Geometry: final body of the model. Coordinates: model frame, mm. Give positions to 0.01 mm unless a question says otherwise; leave off trailing zeros. Write each loop counter-clockwise with the first axis right and the second up, starting at its lowest first coordinate (ties: lowest second). Pieces come first, ordered by that corner, then holes.
```python
from build123d import *

# Parameters (mm, degrees)
BOSS_EXTRUDE1_DEPTH = 5
SKETCH2_W           = 10
SKETCH2_H           = 4
BOSS_EXTRUDE2_DEPTH = 80
FILLET1_R           = 10


with BuildPart() as part:
    # Sketch1 → Boss-Extrude1 (new, symmetric)
    with BuildSketch(Plane(origin=(0, 0, 0), x_dir=(0, 0, -1), z_dir=(1, 0, 0))):
        with BuildLine():
            Line((-75.25, 40), (160.25, 40))
            ThreePointArc((160.25, 40), (166.57455532, 38.973665961), (172.25, 36))
            Line((172.25, 36), (-87.25, 36))
            ThreePointArc((-87.25, 36), (-81.57455532, 38.973665961), (-75.25, 40))
        make_face()
    extrude(amount=BOSS_EXTRUDE1_DEPTH, both=True)

    # Sketch2 → Boss-Extrude2 (add, symmetric)
    with BuildSketch(Plane(origin=(0, 0, 0), x_dir=(0, 0, -1), z_dir=(1, 0, 0))):
        with Locations((42.5, 38)):
            Rectangle(SKETCH2_W, SKETCH2_H)
    extrude(amount=BOSS_EXTRUDE2_DEPTH, both=True)

    # Fillet1
    fillet1_edges = [part.edges().sort_by_distance(p)[0] for p in [
        (-5, 38, -47.5),
        (-5, 38, -37.5),
        (5, 38, -37.5),
        (5, 38, -47.5),
    ]]
    fillet(fillet1_edges, radius=FILLET1_R)


solid = part.part
```
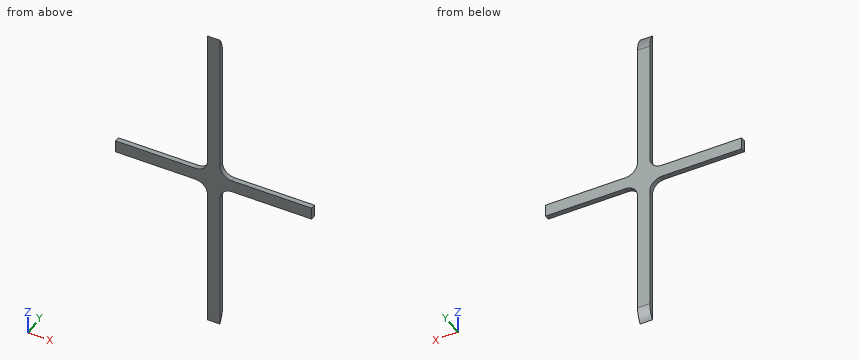
Item 1: Section A-A, the plane y = 36.9. Return the cut outline in (x, z).
Found:
outline: (-80, -47.5) - (-15, -47.5) arc R10 cw to (-5, -57.5) - (-5, -170.95) - (5, -170.95) - (5, -57.5) arc R10 cw to (15, -47.5) - (80, -47.5) - (80, -37.5) - (15, -37.5) arc R10 cw to (5, -27.5) - (5, 85.95) - (-5, 85.95) - (-5, -27.5) arc R10 cw to (-15, -37.5) - (-80, -37.5) - close
Item 2: Section B-B, the plane x = -49.5. Return the cut outline in (y, z), plus the area to 3 significant figures.
Found:
outline: (36, -47.5) - (40, -47.5) - (40, -37.5) - (36, -37.5) - close
area: 40.0 mm2
Item 3: Section C-C, the plane z = -109.5. Return the cut outline in (x, y), plus the area to 3 significant figures.
Found:
outline: (-5, 36) - (5, 36) - (5, 40) - (-5, 40) - close
area: 40.0 mm2
Item 4: Line query: L1, parallel to X at y = 38.45, z = 70; L2, parallel to Z at x = 58.5, y = 36.2; L3, parallel to X at y = 37.5, z = -48.5. Output: solid intervals per line, ascending.
Found:
L1: x = -5 to 5
L2: z = -47.5 to -37.5
L3: x = -10.64 to 10.64
Item 5: Pin query (flat end, axial travel): pin 1 Ø1.5 at (x, y) = (-51.5, 39.5) entering from +Z. Return the tip coordinate at first contact, or that it passes through.
Found:
pin 1: stops at z = -37.5
